Design review of the part shown in the three views and the two pictorial views. Dimensions are in mm from the part's minimum x, y and z. A direction names the side the tool comes from. Give positions to 0.01 mm unless a question says otherwise; leave off trailing zeros. Order: outer loops, then holes, each group sorted by start corner. A loop starts at its lowest first (then second) coordinate and runs counter-clockwise, first axis right, second up. Notation, with made-up numbers: (-8.5, 28.5) -> (28.5, 28.5) arc R12 cw to (28.5, 38.5) -> close; hole circle Ø4 at (-26.75, 30.5). An arc over 180 degrees is marked (long way). Answer in a Markdown table with one row per item. Add a question column.
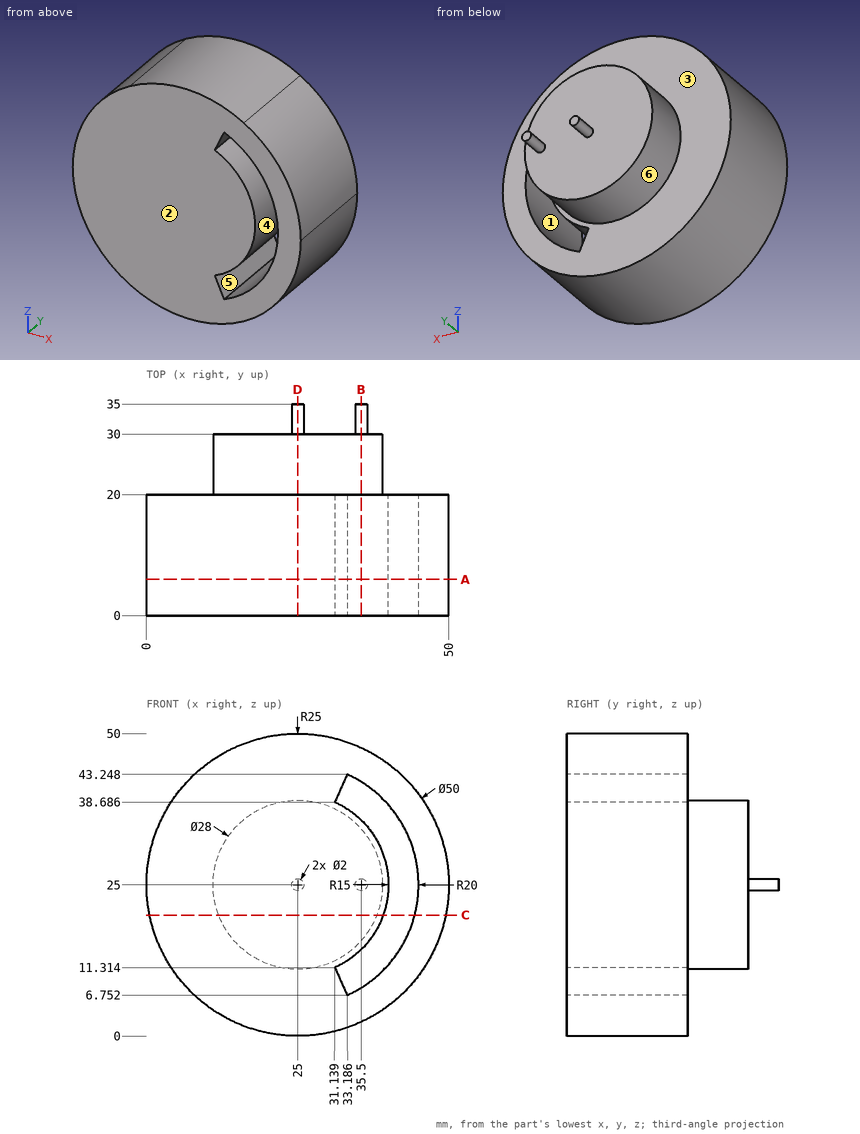
1) Add section D-D, the plane x = 25. Write out the cut boundary in (y, z).
2) Add section C-C, the plane z = 20. Write out the cut boundary in (x, y) (1 decimal).
3) Add section B-B, the plane x = 35.5. Write out the cut boundary in (y, z), and give its area (3 significant figures).
4) Clearance check with flat-ended pins moving along their axes: P1, Ø5, axis at x = 41.5, z = 27, coming from the +Y side; P2, Ø15, axis at x = 34, z = 29.5, coming from the +Y side; P3, Ø2, axis at x = 31, z = 37.5, coming from the +Y side; P4, Ø10, axis at x = 9, y = 6, coming from the +Z side. State where each tip first meets the part, or that it passes through.
5) Mouldability with a two-part tool opening along X and no side actions: class the marked faces 3, 4, 5 and 6 as +X half, -X half, draft (parallel to the pull), parting line (faces both ways), or undercut.
6) Machinability: for the marked faces 1 and 2, which of the approach directions +Z, -Z, +X, -X, +Y, -Y give a long, thin tool a straight path to every point of the face, cutting with its end or side? Answer none if there is none.
7) For L1, parallel to Z at x = 32, y = 14.5 (1 decimal); L2, parallel to Z at x = 35, y = 16; L3, parallel to Y at x = 24, z = 38, list the stretches that pass through material, from the lowest coordinate up.
8) Add section A-A, the plane y = 6. Write out the cut boundary in (x, z).
Verdict:
| question | item | result |
|---|---|---|
| 1 | outline | (0, 0) -> (20, 0) -> (20, 11) -> (30, 11) -> (30, 24) -> (35, 24) -> (35, 26) -> (30, 26) -> (30, 39) -> (20, 39) -> (20, 50) -> (0, 50) -> close |
| 2 | outline | (0.5, 0) -> (39.1, 0) -> (39.1, 20) -> (38.1, 20) -> (38.1, 30) -> (11.9, 30) -> (11.9, 20) -> (0.5, 20) -> close; (44.4, 0) -> (49.5, 0) -> (49.5, 20) -> (44.4, 20) -> close |
| 3 | outline | (0, 2.31) -> (20, 2.31) -> (20, 7.98) -> (0, 7.98) -> close; (0, 14.29) -> (20, 14.29) -> (20, 15.74) -> (30, 15.74) -> (30, 24) -> (35, 24) -> (35, 26) -> (30, 26) -> (30, 34.26) -> (20, 34.26) -> (20, 35.71) -> (0, 35.71) -> close; (0, 42.02) -> (20, 42.02) -> (20, 47.69) -> (0, 47.69) -> close |
| 3 | area | 850 mm2 |
| 4 | P1 | stops at y = 20 |
| 4 | P2 | stops at y = 35 |
| 4 | P3 | stops at y = 30 |
| 4 | P4 | stops at z = 47.45 |
| 5 | face 3 | draft |
| 5 | face 4 | undercut |
| 5 | face 5 | undercut |
| 5 | face 6 | parting line |
| 6 | face 1 | +Y, -Y |
| 6 | face 2 | +Z, -Z, +X, -X, -Y |
| 7 | L1 | z = 1 to 9.4, 11.7 to 38.3, 40.6 to 49 |
| 7 | L2 | z = 2.09 to 7.68, 13.82 to 36.18, 42.32 to 47.91 |
| 7 | L3 | y = 0 to 30 |
| 8 | outline | circle Ø50 at (25, 25); hole (31.14, 11.31) -> (33.19, 6.75) arc R20 ccw to (33.19, 43.25) -> (31.14, 38.69) arc R15 cw to start |
